Here's the drawing with two shaded views (mm, measured from the low corner). I have some questions. A direction names the side the tool comes from. Round coordinates to 2 decimals unless told otherwise and drop trailing zeros. Loops run counter-clockwise (first coordinate to the right, second up) from the corner with the lowest first, then second, coordinate; pieces in that order, holes last. Notation, with made-up numbers: (22.25, -27) - (32.25, -27) arc R30 cw to (32.25, 5) - close; hole circle Ø2 at (28.5, 81.5). An arc over 180 degrees is marked (long way). Answer as CSV lines item,"result".
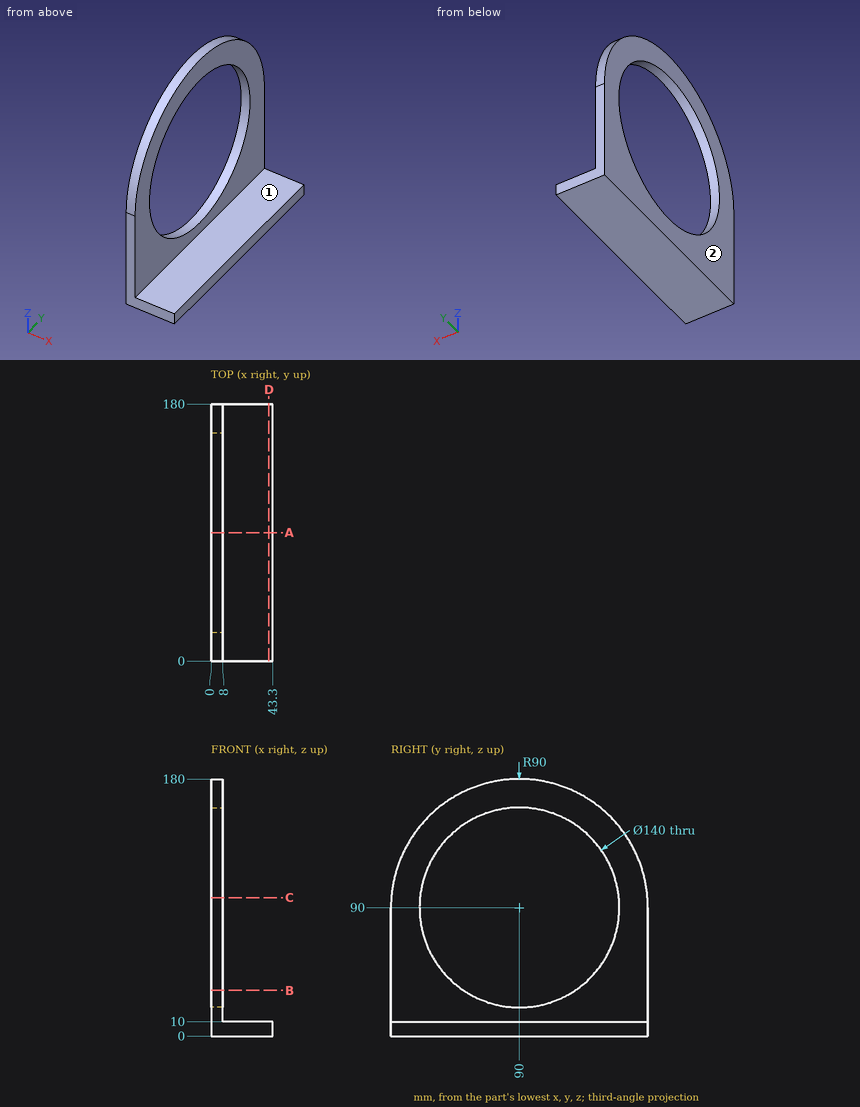
Q1. Imagine slicing it at C-C (z = 97). Write out the boundary of the cut face in (x, y).
Checks:
outline,"(0, 0.27) - (8, 0.27) - (8, 20.35) - (0, 20.35) - close; (0, 159.65) - (8, 159.65) - (8, 179.73) - (0, 179.73) - close"
Q2. If I drill on line 1 along Y through (x, z) = (2.75, 90); line 2 along Z through (x, y) = (25, 85.5); line 3 along X through (y, z) = (160.5, 11.5), over which ranges is the centre line in solid material (lowest first)? Write a range as [from, to].
Checks:
line 1,"[0, 20], [160, 180]"
line 2,"[0, 10]"
line 3,"[0, 8]"
Q3. On a 3-axis mill with a long thin cutter (end or side, diameter ignored), from which of +Z, -Z, +X, -X, +Y, -Y can I reach the whole of each face in a straight line? I mean the marked faces 1 and 2. Say none if no direction works.
Checks:
face 1,"+Z, +X, +Y, -Y"
face 2,"+Z, -Z, -X, +Y, -Y"
Q4. Imagine slicing it at A-A (y = 90). Write out the boundary of the cut face in (x, z), then the cut area to 3 significant figures.
Checks:
outline,"(0, 0) - (43.3, 0) - (43.3, 10) - (8, 10) - (8, 20) - (0, 20) - close; (0, 160) - (8, 160) - (8, 180) - (0, 180) - close"
area,"673 mm²"
Q5. Imagine slicing it at B-B (z = 32). Write out the boundary of the cut face in (x, y), then the cut area to 3 significant figures.
Checks:
outline,"(0, 0) - (8, 0) - (8, 50.81) - (0, 50.81) - close; (0, 129.19) - (8, 129.19) - (8, 180) - (0, 180) - close"
area,"813 mm²"
Q6. I'm going to push flat-ended pins straight in: pin 1 Ø8 at (x, y) = (31.5, 128) entering from +Z; pin 2 Ø10 at (y, z) = (71, 152.5) entering from +X; pin 3 Ø2 at (x, z) = (8.5, 131.5) entering from -Y. Where does each tip first touch, or does it pass through?
Checks:
pin 1,"z = 10"
pin 2,"x = 8"
pin 3,"y = 9.7"
Q7. Imagine slicing it at D-D (x = 40.5). Write out the boundary of the cut face in (y, z).
Checks:
outline,"(0, 0) - (180, 0) - (180, 10) - (0, 10) - close"
